Part model, mm, in its own coordinate system. A direction names the side the tool comes from. Round coordinates to 2 decimals unless told otherwise and drop trailing zeros. Loops run counter-clockwise (first coordinate to the right, second up) from the corner with the lowest first, then second, coordinate; pieces in that order, holes last. Notation, with made-up numbers: M 35,55 L 67,55 A21 cw 67,59 Z; hole C 43.25,-39 d7. An arc over 180 degrees is marked long. Put each result on its own line as item: value. Start each with the question number.
```python
from build123d import *

# Parameters (mm, degrees)
SKETCH1_R           = 7.5
BOSS_EXTRUDE1_DEPTH = 45
BOSS_EXTRUDE2_DEPTH = 6
SKETCH3_R           = 5.25
SKETCH3_R_2         = 4.25
SKETCH3_R_3         = 1.6
CUT_EXTRUDE1_DEPTH  = 7
FILLET1_R           = 5
SKETCH4_R           = 5.1
CUT_EXTRUDE2_DEPTH  = 2
SKETCH5_R           = 12.5
SKETCH5_R_2         = 1.6
CUT_EXTRUDE3_DEPTH  = 46.0000001
CUT_EXTRUDE4_REACH  = 124
SKETCH6_W           = 40
SKETCH6_H           = 25
CUT_EXTRUDE5_REACH  = 124
SKETCH7_R           = 2.55
BOSS_EXTRUDE3_DEPTH = 28
FILLET2_R           = 2
BOSS_EXTRUDE4_DEPTH = 20
FILLET3_R           = 1.2


with BuildPart() as part:
    # Sketch1 → Boss-Extrude1 (new body)
    with BuildSketch(Plane(origin=(0, 0, 0), x_dir=(1, 0, 0), z_dir=(0, 1, 0))):
        with BuildLine():
            ThreePointArc((-47.647058368, -36.465844689), (-41.21916632, -48.520286728), (-39, -62))
            Line((-39, -62), (39, -62))
            ThreePointArc((39, -62), (41.21916632, -48.520286728), (47.647058368, -36.465844689))
            ThreePointArc((47.647058368, -36.465844689), (0, 60), (-47.647058368, -36.465844689))
        make_face()
        with Locations((-33.587572106, -33.587572106)):
            Circle(SKETCH1_R, mode=Mode.SUBTRACT)
        with Locations((33.587572106, -33.587572106)):
            Circle(SKETCH1_R, mode=Mode.SUBTRACT)
        with Locations((-33.587572106, 33.587572106)):
            Circle(SKETCH1_R, mode=Mode.SUBTRACT)
        with BuildLine():
            Line((30, -54), (-30, -54))
            Line((-30, -54), (-30, -48.466483264))
            ThreePointArc((-30, -48.466483264), (-33.435692219, -46.163345696), (-36.695320422, -43.617123463))
            ThreePointArc((-36.695320422, -43.617123463), (-33.334442408, -44.084520489), (-30, -43.455668497))
            ThreePointArc((-30, -43.455668497), (-28.91848754, -24.182804735), (-43.617123463, -36.695320422))
            ThreePointArc((-43.617123463, -36.695320422), (-57, 0), (-43.617123463, 36.695320422))
            ThreePointArc((-43.617123463, 36.695320422), (-26.162950904, 26.162950904), (-36.695320422, 43.617123463))
            ThreePointArc((-36.695320422, 43.617123463), (0, 57), (36.695320422, 43.617123463))
            ThreePointArc((36.695320422, 43.617123463), (26.162950904, 26.162950904), (43.617123463, 36.695320422))
            ThreePointArc((43.617123463, 36.695320422), (57, 0), (43.617123463, -36.695320422))
            ThreePointArc((43.617123463, -36.695320422), (28.91848754, -24.182804735), (30, -43.455668497))
            ThreePointArc((30, -43.455668497), (33.334442408, -44.084520489), (36.695320422, -43.617123463))
            ThreePointArc((36.695320422, -43.617123463), (33.435692219, -46.163345696), (30, -48.466483264))
            Line((30, -48.466483264), (30, -54))
        make_face(mode=Mode.SUBTRACT)
        with Locations((33.587572106, 33.587572106)):
            Circle(SKETCH1_R, mode=Mode.SUBTRACT)
        with BuildLine():
            Line((30, -43.455668497), (30, -48.466483264))
            ThreePointArc((30, -48.466483264), (33.435692219, -46.163345696), (36.695320422, -43.617123463))
            ThreePointArc((36.695320422, -43.617123463), (33.334442408, -44.084520489), (30, -43.455668497))
        make_face()
        with BuildLine():
            ThreePointArc((-36.695320422, -43.617123463), (-33.435692219, -46.163345696), (-30, -48.466483264))
            Line((-30, -48.466483264), (-30, -43.455668497))
            ThreePointArc((-30, -43.455668497), (-33.334442408, -44.084520489), (-36.695320422, -43.617123463))
        make_face()
    extrude(amount=BOSS_EXTRUDE1_DEPTH)

    # Sketch2 → Boss-Extrude2 (add)
    with BuildSketch(Plane.XZ):
        with BuildLine():
            Line((39, 62), (-39, 62))
            ThreePointArc((-39, 62), (-41.21916632, 48.520286728), (-47.647058368, 36.465844689))
            ThreePointArc((-47.647058368, 36.465844689), (0, -60), (47.647058368, 36.465844689))
            ThreePointArc((47.647058368, 36.465844689), (41.21916632, 48.520286728), (39, 62))
        make_face()
    extrude(amount=-BOSS_EXTRUDE2_DEPTH)

    # Sketch3 → Cut-Extrude1 (cut, through all)
    with BuildSketch(Plane(origin=(0, 6, 0), x_dir=(1, 0, 0), z_dir=(0, 1, 0))):
        with Locations((-33.587572106, 33.587572106)):
            Circle(SKETCH3_R)
        with Locations((33.587572106, 33.587572106)):
            Circle(SKETCH3_R)
        with Locations((33.587572106, -33.587572106)):
            Circle(SKETCH3_R)
        with Locations((-33.587572106, -33.587572106)):
            Circle(SKETCH3_R)
        with Locations((0, -33)):
            Circle(SKETCH3_R_2)
        with Locations((-5.75, -27.25)):
            Circle(SKETCH3_R_3)
        with Locations((5.75, -27.25)):
            Circle(SKETCH3_R_3)
        with Locations((5.75, -38.75)):
            Circle(SKETCH3_R_3)
        with Locations((-5.75, -38.75)):
            Circle(SKETCH3_R_3)
    extrude(amount=-CUT_EXTRUDE1_DEPTH, mode=Mode.SUBTRACT)

    # Fillet1
    fillet1_edges = [part.edges().sort_by_distance(p)[0] for p in [
        (43.617123463, 25.5, 36.695320422),
        (43.617123463, 25.5, -36.695320422),
        (36.695320422, 25.5, -43.617123463),
        (-36.695320422, 25.5, -43.617123463),
        (-43.617123463, 25.5, -36.695320422),
        (-43.617123463, 25.5, 36.695320422),
    ]]
    fillet(fillet1_edges, radius=FILLET1_R)

    # Sketch4 → Cut-Extrude2 (cut)
    with BuildSketch(Plane(origin=(0, 6, 0), x_dir=(1, 0, 0), z_dir=(0, 1, 0))):
        with Locations((0, -33)):
            Circle(SKETCH4_R)
    extrude(amount=-CUT_EXTRUDE2_DEPTH, mode=Mode.SUBTRACT)

    # Sketch5 → Cut-Extrude3 (cut, through all)
    with BuildSketch(Plane.XZ):
        with Locations((0, -10)):
            Circle(SKETCH5_R)
        with Locations((15.5, 5.5)):
            Circle(SKETCH5_R_2)
        with Locations((-15.5, 5.5)):
            Circle(SKETCH5_R_2)
        with Locations((-15.5, -25.5)):
            Circle(SKETCH5_R_2)
        with Locations((15.5, -25.5)):
            Circle(SKETCH5_R_2)
    extrude(amount=-CUT_EXTRUDE3_DEPTH, mode=Mode.SUBTRACT)

    # Sketch6 → Cut-Extrude4 (cut, up to next)
    with BuildSketch(Plane.XY.offset(62), mode=Mode.PRIVATE) as cut_extrude4_sk1:
        with Locations((0, 20.5)):
            Rectangle(SKETCH6_W, SKETCH6_H)
    cut_extrude4_tool1 = extrude(cut_extrude4_sk1.sketch, amount=-CUT_EXTRUDE4_REACH, mode=Mode.PRIVATE) & part.part
    add(cut_extrude4_tool1.solids().sort_by_distance((0, 20.5, 62))[0], mode=Mode.SUBTRACT)

    # Sketch7 → Cut-Extrude5 (cut, up to next)
    with BuildSketch(Plane.XY.offset(62), mode=Mode.PRIVATE) as cut_extrude5_sk1:
        with Locations((-25.5, 10.5)):
            Circle(SKETCH7_R)
    cut_extrude5_tool1 = extrude(cut_extrude5_sk1.sketch, amount=-CUT_EXTRUDE5_REACH, mode=Mode.PRIVATE) & part.part
    add(cut_extrude5_tool1.solids().sort_by_distance((-25.5, 10.5, 62))[0], mode=Mode.SUBTRACT)
    # Sketch7 → Cut-Extrude5 (cut, up to next)
    with BuildSketch(Plane.XY.offset(62), mode=Mode.PRIVATE) as cut_extrude5_sk2:
        with Locations((25.5, 10.5)):
            Circle(SKETCH7_R)
    cut_extrude5_tool2 = extrude(cut_extrude5_sk2.sketch, amount=-CUT_EXTRUDE5_REACH, mode=Mode.PRIVATE) & part.part
    add(cut_extrude5_tool2.solids().sort_by_distance((25.5, 10.5, 62))[0], mode=Mode.SUBTRACT)
    # Sketch7 → Cut-Extrude5 (cut, up to next)
    with BuildSketch(Plane.XY.offset(62), mode=Mode.PRIVATE) as cut_extrude5_sk3:
        with Locations((25.5, 28.5)):
            Circle(SKETCH7_R)
    cut_extrude5_tool3 = extrude(cut_extrude5_sk3.sketch, amount=-CUT_EXTRUDE5_REACH, mode=Mode.PRIVATE) & part.part
    add(cut_extrude5_tool3.solids().sort_by_distance((25.5, 28.5, 62))[0], mode=Mode.SUBTRACT)
    # Sketch7 → Cut-Extrude5 (cut, up to next)
    with BuildSketch(Plane.XY.offset(62), mode=Mode.PRIVATE) as cut_extrude5_sk4:
        with Locations((-25.5, 28.5)):
            Circle(SKETCH7_R)
    cut_extrude5_tool4 = extrude(cut_extrude5_sk4.sketch, amount=-CUT_EXTRUDE5_REACH, mode=Mode.PRIVATE) & part.part
    add(cut_extrude5_tool4.solids().sort_by_distance((-25.5, 28.5, 62))[0], mode=Mode.SUBTRACT)

    # Sketch8 → Boss-Extrude3 (add)
    with BuildSketch(Plane(origin=(0, 6, 0), x_dir=(1, 0, 0), z_dir=(0, 1, 0))):
        with BuildLine():
            Line((-36.587572106, 23.525266208), (-36.587572106, -23.525266208))
            ThreePointArc((-36.587572106, -23.525266208), (-33.587572106, -23.087572106), (-30.587572106, -23.525266208))
            Line((-30.587572106, -23.525266208), (-30.587572106, 23.525266208))
            ThreePointArc((-30.587572106, 23.525266208), (-33.587572106, 23.087572106), (-36.587572106, 23.525266208))
        make_face()
        with BuildLine():
            Line((30.587572106, 23.525266208), (30.587572106, -23.525266208))
            ThreePointArc((30.587572106, -23.525266208), (33.587572106, -23.087572106), (36.587572106, -23.525266208))
            Line((36.587572106, -23.525266208), (36.587572106, 23.525266208))
            ThreePointArc((36.587572106, 23.525266208), (33.587572106, 23.087572106), (30.587572106, 23.525266208))
        make_face()
    extrude(amount=BOSS_EXTRUDE3_DEPTH)

    # Fillet2
    fillet2_edges = [part.edges().sort_by_distance(p)[0] for p in [
        (-30.587572106, 20, -23.525266208),
        (-36.587572106, 20, -23.525266208),
        (-36.587572106, 20, 23.525266208),
        (-30.587572106, 20, 23.525266208),
        (30.587572106, 20, 23.525266208),
        (36.587572106, 20, 23.525266208),
        (36.587572106, 20, -23.525266208),
        (30.587572106, 20, -23.525266208),
        (30, 25.5, 43.455668497),
        (-30, 25.5, 43.455668497),
    ]]
    fillet(fillet2_edges, radius=FILLET2_R)

    # Sketch9 → Boss-Extrude4 (add)
    with BuildSketch(Plane(origin=(0, 6, 0), x_dir=(1, 0, 0), z_dir=(0, 1, 0))):
        with BuildLine():
            Line((-23.525266208, 30.587572106), (23.525266208, 30.587572106))
            ThreePointArc((23.525266208, 30.587572106), (23.087572106, 33.587572106), (23.525266208, 36.587572106))
            Line((23.525266208, 36.587572106), (-23.525266208, 36.587572106))
            ThreePointArc((-23.525266208, 36.587572106), (-23.087572106, 33.587572106), (-23.525266208, 30.587572106))
        make_face()
    extrude(amount=BOSS_EXTRUDE4_DEPTH)

    # Fillet3
    fillet3_edges = [part.edges().sort_by_distance(p)[0] for p in [
        (20, 33, 58),
        (20, 8, 58),
        (-20, 8, 58),
        (-20, 33, 58),
    ]]
    fillet(fillet3_edges, radius=FILLET3_R)


solid = part.part
```
1. Which spindle directions (+Z, -Z, +X, -X, +Y, -Y) get a long thin tool onto all of the face, cutting with end or side? Do faces 4 (the cylindrical face through (13.9, 2.96, 5.57)), 5 (the flat face through (-20, 20, 58)), 6 (the flat face through (-30.588, 20, 0)). Say none if no direction does.
2. Cut at A-A, the plane x = 0. Give the cut face in (y, z), and give its area (3 significant figures).
3. Cut at B-B, the plane z = 5.5. Give the cut face in (x, y).
4. Wall check: L1, parallel to Y at x = 25.5, z = 57.25; L2, parallel to X at y = 21, z = 1; L3, parallel to Z at x = 34.5, y = 14. Give the ranges that are in metal, low to high.
5. Cut at D-D, the plane z = 48.5. Give the cut face in (x, y), and give its area (3 significant figures).
6. Mould opens along Y. For faces 1 (the flat face through (-39, 6, -35)), 2 (the flat face through (0, 33, 58)), 3 (the cylindrical face through (41.16, 22.18, 48.7)) say: released by +Y, released by -Y, zero draft, split by the parting line, or undercut.
7. Drop flat-ended pins along their axis: pin 1 (4 mm diameter, centred on x = -39, y = 19, fed in from -Z); pin 2 (5 mm diameter, centred on x = -30, y = 30.5, fed in from -Z); pin 3 (5 mm diameter, centred on y = 7, z = -28.5, fed in from +X); pin 4 (2.5 mm diameter, centred on x = 5.75, z = 38.75, fed in from +Y). Give the stop position or say it passes through.
8. Cut at C-C, the plane y = 40.5. Give the number of separate pieces and of enclosed holes in the cut face, and give its area (3 significant figures).
Results list:
1. face 4: +Y, -Y
1. face 5: +Z
1. face 6: +Y
2. outline: M 0,-60 L 45,-60 L 45,-57 L 6,-57 L 6,-36.59 L 26,-36.59 L 26,-30.59 L 6,-30.59 L 6,-22.5 L 0,-22.5 Z; M 0,2.5 L 6,2.5 L 6,27.9 L 4,27.9 L 4,28.75 L 0,28.75 Z; M 0,37.25 L 4,37.25 L 4,38.1 L 6,38.1 L 6,54 L 8,54 L 8,62 L 0,62 Z; M 33,54 L 45,54 L 45,62 L 33,62 Z
2. area: 877 mm^2
3. outline: M -59.75,0 L -17.1,0 L -17.1,6 L -30.59,6 L -30.59,34 L -36.59,34 L -36.59,6 L -56.73,6 L -56.73,45 L -59.75,45 Z; M -13.9,0 L 13.9,0 L 13.9,6 L -13.9,6 Z; M 17.1,0 L 59.75,0 L 59.75,45 L 56.73,45 L 56.73,6 L 36.59,6 L 36.59,34 L 30.59,34 L 30.59,6 L 17.1,6 Z
4. L1: y = 0 to 7.95, 13.05 to 25.95, 31.05 to 45
4. L2: x = -59.99 to -56.99, -36.59 to -30.59, 30.59 to 36.59, 56.99 to 59.99
4. L3: z = -49.09 to -41.03, -26.14 to 26.14, 41.03 to 62
5. outline: M -41.23,0 L 41.23,0 L 41.23,45 L 30,45 L 30,6 L -30,6 L -30,45 L -41.23,45 Z
5. area: 1,370 mm^2
6. face 1: released by +Y
6. face 2: undercut
6. face 3: zero draft
7. pin 1: stops at z = -47.23
7. pin 2: stops at z = -53.33
7. pin 3: stops at x = 54.07
7. pin 4: passes through
8. separate pieces: 1
8. enclosed holes: 5
8. area: 2,500 mm^2
